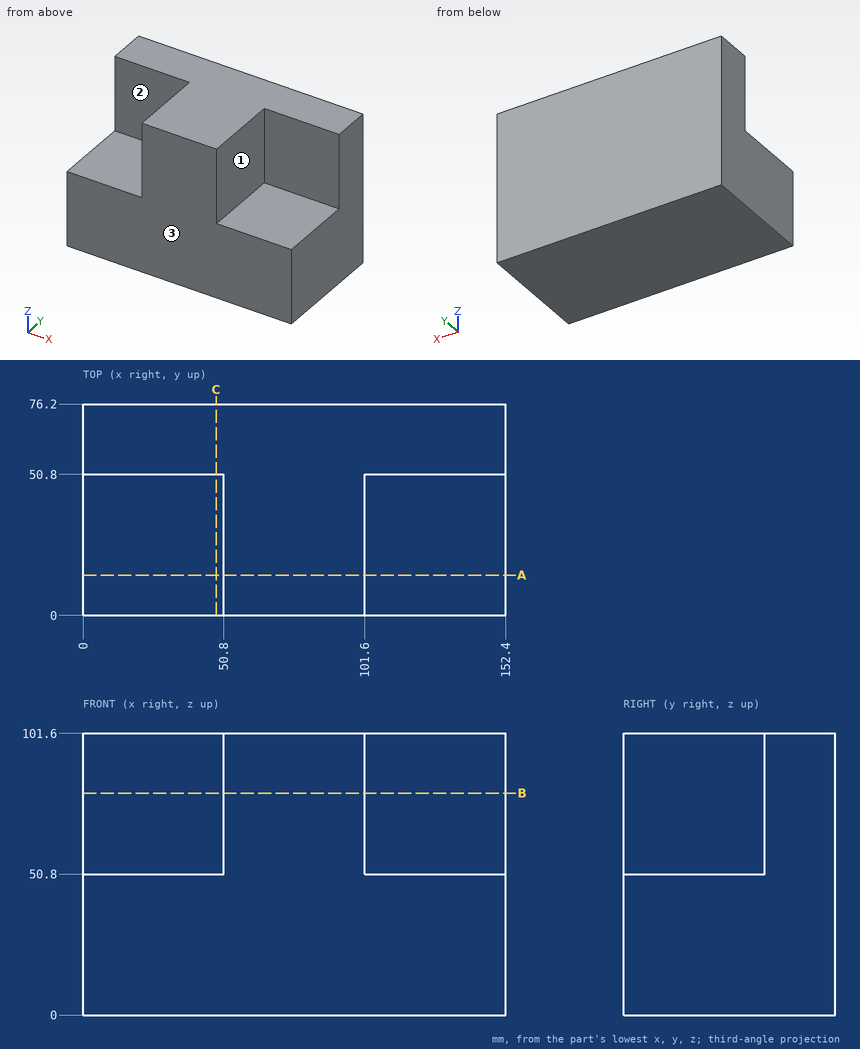
Input: dimensioned drawing with shaded views. Units: mm. Origin: part minimum x, y, z. A direction names the side the tool comes from. Coordinates: 2 decimals unless noted, no trailing zeros. Order: outer loops, then holes, each group sorted by start corner. A loop starts at its lowest first (then second) coordinate and runs counter-clockwise, first axis right, second up. Notation, with made-up numbers: (-20.5, 20.25) -> (-1.5, 20.25) arc R26 ccw to (-1.5, 51.25) -> close; hole circle Ø9 at (79, -10). An arc over 180 degrees is marked (long way). Use CSV: the item, a comma, the result in double quotes.
1) Section C-C on x = 48. Output: boundary loops of the cut face in (y, z), then the cut area to 3 significant figures.
Findings:
outline,"(0, 0) -> (76.2, 0) -> (76.2, 101.6) -> (50.8, 101.6) -> (50.8, 50.8) -> (0, 50.8) -> close"
area,"5,160 mm^2"
2) Pin query (flat end, axial travel): pin 1 Ø15 at (x, y) = (114.5, 25) entering from +Z; pin 2 Ø4 at (x, z) = (111.5, 68.5) entering from -Y. Return the tip coordinate at first contact, or that it passes through.
Findings:
pin 1,"stops at z = 50.8"
pin 2,"stops at y = 50.8"
3) Access query for the marked faces 1, 2 and 3. Directions: +Z, -Z, +X, -X, +Y, -Y. A direction counts if a zero-diameter tool reaches every point of the face in a straight line with its end or side. Return the directions, or none.
Findings:
face 1,"+Z, +X, -Y"
face 2,"+Z, -X, -Y"
face 3,"+Z, -Z, +X, -X, -Y"
4) Section B-B on z = 80. Output: boundary loops of the cut face in (x, y), then the cut area to 3 significant figures.
Findings:
outline,"(0, 50.8) -> (50.8, 50.8) -> (50.8, 0) -> (101.6, 0) -> (101.6, 50.8) -> (152.4, 50.8) -> (152.4, 76.2) -> (0, 76.2) -> close"
area,"6,450 mm^2"
5) Line query: line 1 (Y direction, x = 107, z = 81.5); line 2 (Z direction, x = 130, y = 41); line 3 (X direction, y = 25, z = 56). Output: solid intervals per line, ascending.
Findings:
line 1,"y = 50.8 to 76.2"
line 2,"z = 0 to 50.8"
line 3,"x = 50.8 to 101.6"
6) Section A-A on y = 14.5. Output: boundary loops of the cut face in (x, z).
Findings:
outline,"(0, 0) -> (152.4, 0) -> (152.4, 50.8) -> (101.6, 50.8) -> (101.6, 101.6) -> (50.8, 101.6) -> (50.8, 50.8) -> (0, 50.8) -> close"
